Study the drawing (mm; zero at the part's minimum x, y, z) and answer. A direction names the side the tool comes from. Coordinates: 2 decimals unless noted, no trailing zeros. Order: outer loops, then holes, each group sorted by start corner. A loop starts at its lowest first (then second) coordinate and runs counter-clockwise, first axis right, second up.
1. A flat-ended cylindrical pin translates along its axis: pin 1 Ø2 at (x, z) = (6.5, 6.5) entering from +Y. Find the tip coordinate at first contact, or state that the pin passes through.
2. Find the intervals of material crossed by probe 1 along Y at (x, z) = (4.25, 9) (3 decimals); probe 2 along X at (y, z) = (1.5, 13.5), in increasing order.
3. Determine the mould class of the marked faces 3, 4 and 5 for opening direction Y: +Y half, -Y half, draft (parallel to the pull), parting line (faces both ways), or undercut.
4. The part is cut by section D-D, the plane y = 13.25. Give the vertices of the cut face in (x, z), then the cut area to 3 significant figures.
5. A tool of negligible diameter and unlimited length cuts with its end or side. For the marked faces 1 and 2, from which of +Z, -Z, +X, -X, +Y, -Y can it reach the whole face along a straight path? Write none if from no direction.
6. The part is cut by section C-C, the plane x = 2. Give the vertices of the cut face in (y, z) (3 decimals), then the cut area to 3 significant figures.
7. The part is cut by section A-A, the plane y = 9. Give the vertices of the cut face in (x, z) (3 decimals).
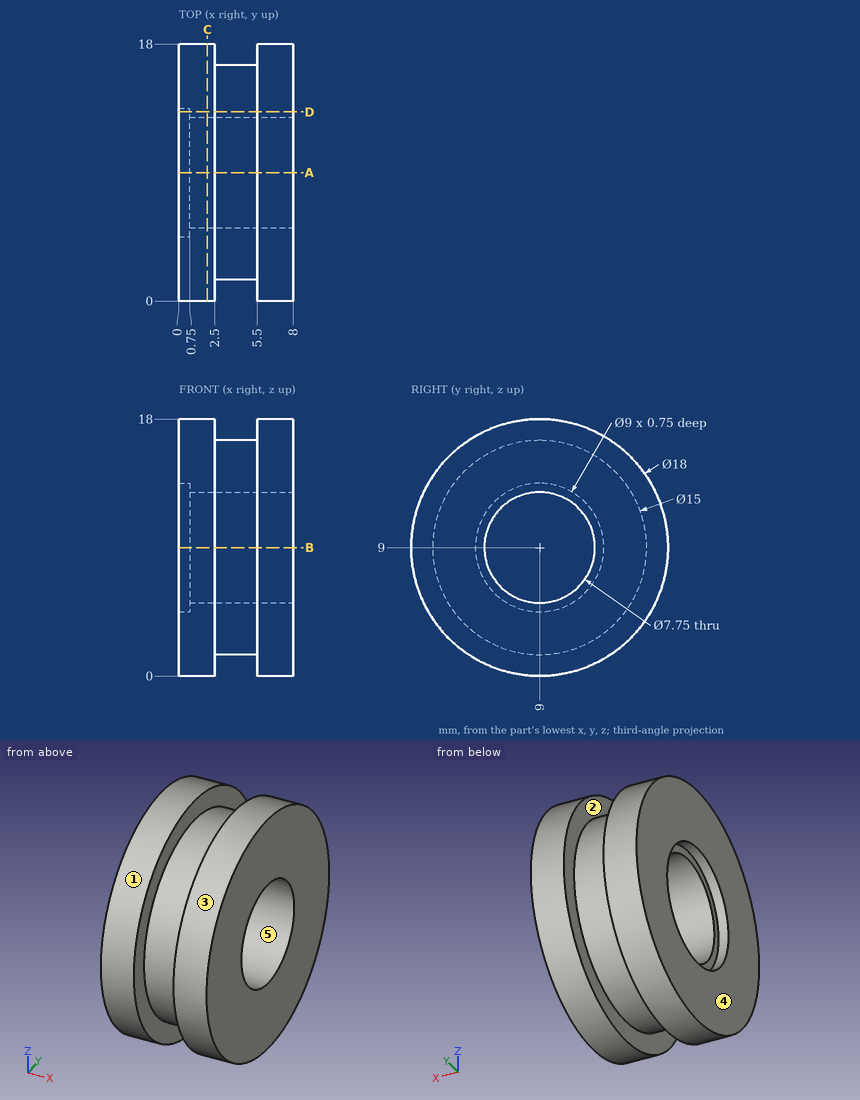
Geometry says:
1. pin 1: stops at y = 17.87
2. probe 1: y = 1.5 to 5.125, 12.875 to 16.5
2. probe 2: x = 0 to 2.5, 5.5 to 8
3. face 3: parting line
3. face 4: draft
3. face 5: undercut
4. outline: (0, 1.07) - (2.5, 1.07) - (2.5, 2.82) - (5.5, 2.82) - (5.5, 1.07) - (8, 1.07) - (8, 16.93) - (5.5, 16.93) - (5.5, 15.18) - (2.5, 15.18) - (2.5, 16.93) - (0, 16.93) - (0, 10.48) - (0.75, 10.48) - (0.75, 7.52) - (0, 7.52) - close
4. area: 114 mm2
5. face 1: +X, -X
5. face 2: none
6. outline: circle Ø18 at (9, 9); hole circle Ø7.75 at (9, 9)
6. area: 207 mm2
7. outline: (0, 0) - (2.5, 0) - (2.5, 1.5) - (5.5, 1.5) - (5.5, 0) - (8, 0) - (8, 5.125) - (0.75, 5.125) - (0.75, 4.5) - (0, 4.5) - close; (0, 13.5) - (0.75, 13.5) - (0.75, 12.875) - (8, 12.875) - (8, 18) - (5.5, 18) - (5.5, 16.5) - (2.5, 16.5) - (2.5, 18) - (0, 18) - close
